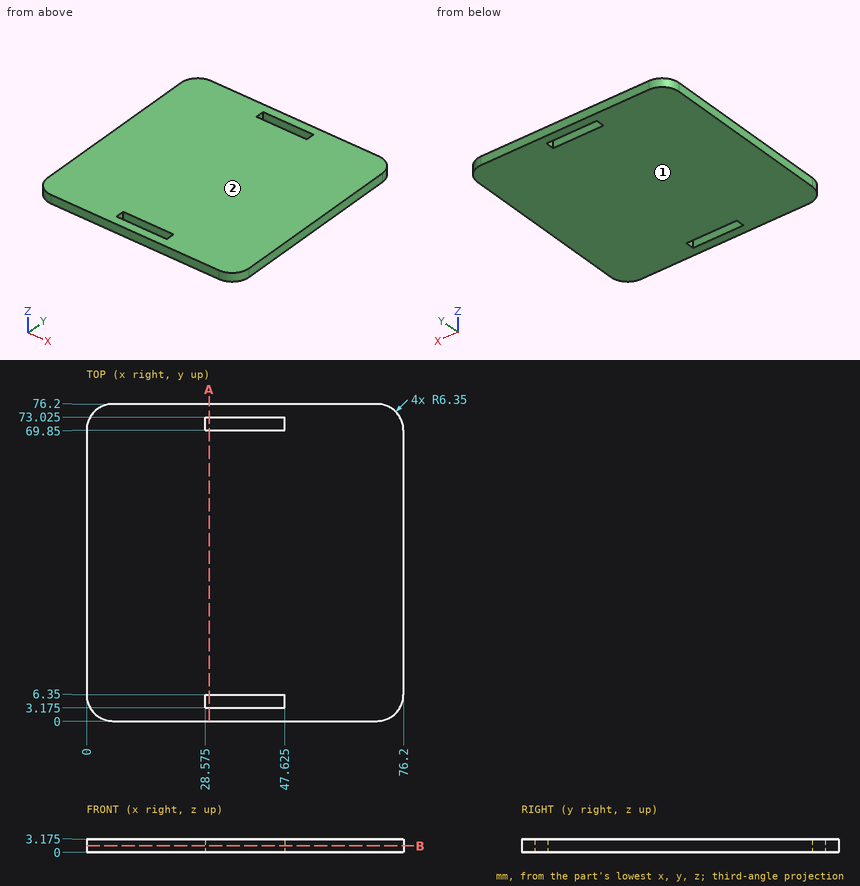
Drawing for the job (mm, zero at the part's lowest x, y, z). Give positions to 0.01 mm unless a question says otherwise; leave off trailing zeros. Loops run counter-clockwise (first coordinate to the right, second up) from the corner with the lowest first, then second, coordinate; pieces in that order, holes last. Notation, with made-up numbers: M -36,-19.75 L 0,-19.75 A29 cw 0,9.25 Z; hole C -10,53 d2. An arc over 180 degrees is marked long. One line per question, with ' | ' between items. Start each with the question number.
1. Flat gauge pins, fed straight in: pin 1 (1.6 mm diameter, centred on y = 4.5, z = 2, fed in from -X); pin 2 (1.6 mm diameter, centred on y = 71, z = 1, fed in from +X). Where does each tip first touch, or does it go through?
2. Saw through at B-B on z = 1.5. Give the cut face in (x, y) (3 decimals).
3. Probe L1, parallel to Y at x = 36, z = 0.45 (3 decimals); L2, parallel to X at y = 72.5, z = 0.9 (3 decimals); L3, parallel to X at y = 5.5, z = 1.65 (3 decimals). List the from-to ranges inside material, lowest first. Write a range as from..to.
4. Two-plate mould, pull along Z, no slides. Class the marked faces 1 and 2: pulls with the +Z half, pulls with the -Z half, needs draft (parallel to the pull), parting line crosses it, or undercut.
5. Saw through at A-A on x = 29.5. Give the cut face in (y, z) (3 decimals), plus the area to 3 significant figures.
Result sheet:
1) pin 1: stops at x = 0.09 | pin 2: stops at x = 76.19
2) outline: M 0,6.35 A6.35 ccw 6.35,0 L 69.85,0 A6.35 ccw 76.2,6.35 L 76.2,69.85 A6.35 ccw 69.85,76.2 L 6.35,76.2 A6.35 ccw 0,69.85 Z; hole M 28.575,3.175 L 47.625,3.175 L 47.625,6.35 L 28.575,6.35 Z; hole M 28.575,69.85 L 47.625,69.85 L 47.625,73.025 L 28.575,73.025 Z
3) L1: y = 0..3.175, 6.35..69.85, 73.025..76.2 | L2: x = 0.579..28.575, 47.625..75.621 | L3: x = 0.057..28.575, 47.625..76.143
4) face 1: pulls with the -Z half | face 2: pulls with the +Z half
5) outline: M 0,0 L 3.175,0 L 3.175,3.175 L 0,3.175 Z; M 6.35,0 L 69.85,0 L 69.85,3.175 L 6.35,3.175 Z; M 73.025,0 L 76.2,0 L 76.2,3.175 L 73.025,3.175 Z | area: 222 mm^2
